```python
from build123d import *

# Parameters (mm, degrees)
SKETCH2_R   = 4.5
SKETCH2_R_2 = 3.5


with BuildPart() as part:
    # Sweep1: sweep along a curve in space
    with BuildLine() as sweep1_path:
        Line((0, 0, 0), (-25, 0, 0))
        Line((0, 0, 0), (65, 13.43503, 34.64823))
        Line((65, 13.43503, 34.64823), (75, 13.43503, 34.64823))
    # Sketch2 → Sweep1 (sweep)
    with BuildSketch(Plane(origin=(0, 0, 0), x_dir=(0, 0, -1), z_dir=(1, 0, 0))):
        Circle(SKETCH2_R)
        Circle(SKETCH2_R_2, mode=Mode.SUBTRACT)
    sweep(path=sweep1_path.line, transition=Transition.RIGHT)


solid = part.part
```
The model under review builds one solid part; all positions refer to its coordinate system, in mm. A direction names the side the tool comes from. Give positions to 0.01 mm unless a question says otherwise; leave off trailing zeros. Write each loop counter-clockwise with the first axis right and the second up, starting at its lowest first coordinate (ties: lowest second). Pieces come first, ordered by that corner, then holes. Notation, with made-up numbers: (-7, 10) -> (-2, 10) arc R31 cw to (-2, 37) -> close; hole circle Ø2 at (-17, 32.5). An arc over 180 degrees is marked (long way). Answer in a Markdown table with one row per item.
1) Mouldability with a two-part tool opening along Z and no side actions: class faces 4 (the cylindrical face through (29.887, 9.153, 20.114)), 5 (the cylindrical face through (30.443, 6.314, 20.178)), 6 (the flat face through (75, 16, 32)) as +Z half, -Z half, draft (parallel to the pull), parting line (faces both ways), or undercut.
Worked answers:
| item | result |
|---|---|
| face 4 | parting line |
| face 5 | undercut |
| face 6 | draft |
2) Clearance check with flat-ended pins moving along their axes: P1, Ø1, axis at x = 63, y = 10.5, coming from the +Z side; P2, Ø12, axis at y = 12.5, z = 13, coming from the +X side; P3, Ø6, axis at x = -10, z = 3.5, coming from the -Y side; P4, Ø8, axis at y = 0, z = 0, coming from the -X side. State where each tip first meets the part, or that it passes through.
Worked answers:
| item | result |
|---|---|
| P1 | z = 37.98 |
| P2 | x = 43.78 |
| P3 | y = -4.47 |
| P4 | x = -25 |
3) For L1, parallel to Y at x = -18.5, z = 0; L2, parallel to Z at x = 38.5, y = 7.25; L3, parallel to Z at x = 32, y = 6.5, list the stretches that pass through material, from the lowest coordinate up. Write a range as [from, to].
Worked answers:
| item | result |
|---|---|
| L1 | [-4.5, -3.5], [3.5, 4.5] |
| L2 | [15.43, 16.58], [24.32, 25.46] |
| L3 | [11.97, 13.1], [20.99, 22.12] |
4) Add section A-A on x = -14. State the section outline as (y, z) points, plus the area to 3 significant figures.
Worked answers:
| item | result |
|---|---|
| outline | circle Ø9 at (0, 0); hole circle Ø7 at (0, 0) |
| area | 25.1 mm² |
5) Tool access review of faces 1 (the cylindrical face through (69.3, 16.2, 38.2)), 2 (the cylindrical face through (-12.086, -1.352, -4.292)), 3 (the flat face through (-25, 4, 0)): name each direction out of +Z, -Z, +X, -X, +Y, -Y from which nothing blocks a thin tool from reaching the whole face with its end or side.
Worked answers:
| item | result |
|---|---|
| face 1 | +X |
| face 2 | -X |
| face 3 | +Z, -Z, -X, +Y, -Y |
